CAD build for the part. Positions are in the model's coordinates, mm. A direction names the side the tool comes from. Coordinates: 2 decimals unless noted, no trailing zeros. Order: outer loops, then holes, each group sorted by start corner. A loop starts at its lowest first (then second) coordinate and runs counter-clockwise, first axis right, second up. Notation, with made-up numbers: (-4, 49) -> (13, 49) arc R17 ccw to (13, 74) -> close; hole circle Ø3 at (-28, 77.25). An arc over 180 degrees is marked (long way). Use one line per item in the form item = value. Start each with the question number.
from build123d import *

# Parameters (mm, degrees)
BOSS_EXTRU_1_DEPTH      = 19
ENL_V_MAT_EXTRU_2_DEPTH = 12
ESQUISSE4_R             = 1.75
ENL_V_MAT_EXTRU_3_DEPTH = 12
ESQUISSE5_R             = 1.25
BOSS_EXTRU_2_DEPTH      = 3


with BuildPart() as part:
    # Esquisse1 → Boss.-Extru.1 (new body)
    with BuildSketch(Plane(origin=(0, 0, 0), x_dir=(1, 0, 0), z_dir=(0, 1, 0))):
        with BuildLine():
            Line((0, 0), (35, 0))
            Line((35, 0), (35, 15))
            Line((35, 15), (0, 15))
            ThreePointArc((0, 15), (-7.5, 7.5), (0, 0))
        make_face()
    extrude(amount=BOSS_EXTRU_1_DEPTH)

    # Esquisse3 → Enlèv. mat.-Extru.2 (cut)
    with BuildSketch(Plane.XY):
        Polygon((6, 19), (29, 19), (29, 16), (35, 16), (35, 3.144779012), (35, 0), (29, 0), (29, 3), (6, 3), (6, 0), (0, 0), (0, 3.824764885), (0, 16), (6, 16), align=None)
    extrude(amount=-ENL_V_MAT_EXTRU_2_DEPTH, mode=Mode.SUBTRACT)

    # Esquisse4 → Enlèv. mat.-Extru.3 (cut)
    with BuildSketch(Plane(origin=(0, 19, 0), x_dir=(1, 0, 0), z_dir=(0, 1, 0))):
        with Locations((32.3, 6)):
            Circle(ESQUISSE4_R)
        with Locations((2.7, 6)):
            Circle(ESQUISSE4_R)
    extrude(amount=-ENL_V_MAT_EXTRU_3_DEPTH, mode=Mode.SUBTRACT)

    # Esquisse5 → Boss.-Extru.2 (add)
    with BuildSketch(Plane.XZ):
        with Locations((23, -6)):
            Circle(ESQUISSE5_R)
    extrude(amount=BOSS_EXTRU_2_DEPTH)


solid = part.part
1) Probe L1, parallel to Z at x = 2.7, y = 18; L2, parallel to X at y = 18.1, z = -6; L3, parallel to Y at x = 19, z = -9.25. List the from-to ranges inside material, lowest first.
2) Cut at A-A on x = 2.7. Give the cut face in (y, z).
3) Drop flat-ended pins along their axis: P1, Ø3, axis at x = 32.3, z = -6, coming from the -Y side; P2, Ø2.5, axis at y = 1, z = -8, coming from the +X side; P3, Ø8, axis at x = -2.5, z = -13.5, coming from the -Y side; P4, Ø0.9, axis at y = 18, z = -5.5, coming from the -X side. Give the stop position or say it passes through.
4) Cut at D-D on y = 11.25. Give the cut face in (x, z).
5) 3-axis set-ups, long thin cutter, end or side, ignore diameter. For faces 1 (the face through (6, 17, -6)), 2 (the face through (3, 17, 0)), 3 (the face through (18, 3, -6)), 4 (the face through (30.6, 16, -4.6)), 5 (the face through (6, 2, -6)): which of +Z, -Z, +X, -X, +Y, -Y reach the whole face in a straight line?
6) Cut at C-C on z = -8.75. Give the cut face in (x, y).
7) Two-plate mould, pull along Z, no slides. Class faces 6 (the face through (0, 8, -6)), 7 (the face through (2.32, 17.52, -4.29)), 8 (the face through (33.917, 17.521, -5.33)), 9 (the face through (24.155, -1.479, -6.479)): released by +Z, released by -Z, zero draft, split by the parting line, or undercut.
8) Cut at B-B on z = -6. Give the cut face in (x, y), then the cut area to 3 significant figures.
Values follow:
q1.L1 = -15 to -7.75, -4.25 to 0
q1.L2 = -7.35 to 0.95, 4.45 to 6, 29 to 30.55, 34.05 to 35
q1.L3 = 0 to 3
q2.outline = (0, -15) -> (19, -15) -> (19, -7.75) -> (16, -7.75) -> (16, -12) -> (0, -12) -> close; (16, -4.25) -> (19, -4.25) -> (19, 0) -> (16, 0) -> close
q3.P1 = through
q3.P2 = 29
q3.P3 = 0
q3.P4 = -7.34
q4.outline = (0, -15) -> (35, -15) -> (35, -12) -> (0, -12) -> (0, 0) arc R7.5 ccw to start
q5.face_1 = +Z, +Y
q5.face_2 = +Z, +X, -X, +Y, -Y
q5.face_3 = +Z, +X, +Y
q5.face_4 = +Z, +X, -Y
q5.face_5 = +Z, -Y
q6.outline = (-7.4, 0) -> (0, 0) -> (0, 16) -> (6, 16) -> (6, 19) -> (-7.4, 19) -> close; (6, 0) -> (29, 0) -> (29, 3) -> (6, 3) -> close; (29, 16) -> (35, 16) -> (35, 19) -> (29, 19) -> close
q7.face_6 = zero draft
q7.face_7 = undercut
q7.face_8 = undercut
q7.face_9 = split by the parting line
q8.outline = (-7.35, 0) -> (0, 0) -> (0, 16) -> (0.95, 16) -> (0.95, 19) -> (-7.35, 19) -> close; (4.45, 16) -> (6, 16) -> (6, 19) -> (4.45, 19) -> close; (6, 0) -> (21.75, 0) -> (21.75, -3) -> (24.25, -3) -> (24.25, 0) -> (29, 0) -> (29, 3) -> (6, 3) -> close; (29, 16) -> (30.55, 16) -> (30.55, 19) -> (29, 19) -> close; (34.05, 16) -> (35, 16) -> (35, 19) -> (34.05, 19) -> close
q8.area = 231 mm^2
